from build123d import *

# Parameters (mm, degrees)
F0_W           = 40
F0_H           = 16
F1_DEPTH       = 12.7
F3_DEPTH       = 3.7
F4_R           = 6
F5_DEPTH       = 6
F6_R           = 8
F7_DEPTH       = 3
F9_D           = 5
F9_CBORE_D     = 9
F9_CBORE_DEPTH = 5


with BuildPart() as f1:
    # F0 (on Top) → F1 (new body)
    with BuildSketch(Plane.XY):
        Rectangle(F0_W, F0_H)
    extrude(amount=F1_DEPTH)

    # F2 (on face) → F3 (cut)
    with BuildSketch(Plane.XY.offset(12.7)):
        with BuildLine():
            ThreePointArc((-8, 8), (0, 0), (8, 8))
            Line((8, 8), (-8, 8))
        make_face()
    extrude(amount=-F3_DEPTH, mode=Mode.SUBTRACT)

    # F4 (on face) → F5 (cut)
    with BuildSketch(Plane.XY.offset(9)):
        with Locations((0, 8)):
            Circle(F4_R)
    extrude(amount=-F5_DEPTH, mode=Mode.SUBTRACT)

    # F6 (on face) → F7 (cut)
    with BuildSketch(Plane.XY.offset(3)):
        with Locations((0, 8)):
            Circle(F6_R)
    extrude(amount=-F7_DEPTH, mode=Mode.SUBTRACT)

    # F9 (through all)
    with Locations(Plane.XZ.offset(8)):
        with Locations((-13, 6), (13, 6)):
            CounterBoreHole(F9_D / 2, F9_CBORE_D / 2, F9_CBORE_DEPTH)


solid = f1.part
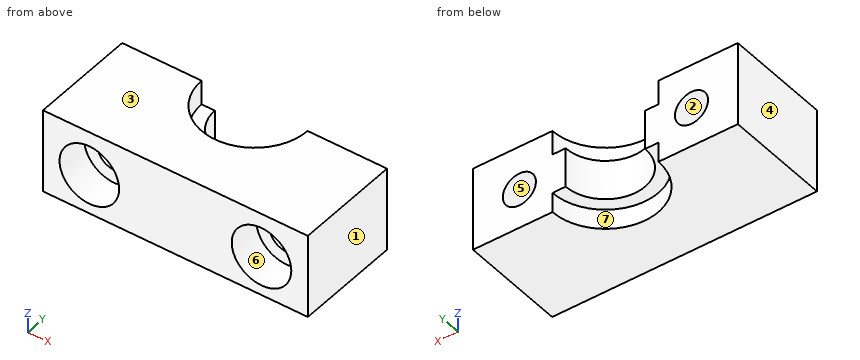
The listing builds one solid part. Answer for the finished solid, in the listing's coordinates (mm). Face numbers are marked on the shaded views. A direction names the side the tool comes from. Coordinates: 2 decimals unless noted, no trailing zeros. Order: outer loops, then holes, each group sorted by start corner. A loop starts at its lowest first (then second) coordinate and runs counter-clockwise, first axis right, second up.
Q1. Which of the six approach directions +Z, -Z, +X, -X, +Y, -Y give full straight-line access (tool end or side, diameter ignored) to the marked faces 5, 6 and 7?
Q2. A cutting plane is placed at A-A, the plane x = -13. Write down the section's boundary in (y, z).
Q3. A cutting plane is placed at D-D, the plane y = -4.25. Write down the section's boundary in (x, z), and give its area (3 significant figures).
Q4. For a pull along X with two mould halves and no side action, classify the marked faces 1, 2, 3 and 4 as pulls with the +X half, pulls with the -X half, needs draft (parallel to the pull), parting line crosses it, or undercut.
Q5. Given P1, Ø2.5, axis at x = 12.5, z = 6.5, coming from the -Y side; P2, Ø2, axis at x = 12.5, y = -3, coming from the -Z side; P3, Ø1.5, axis at x = -1.5, z = 10, coming from the +Y side; P4, Ø4.5, axis at x = -13.5, z = 5.5, coming from the -Y side, each flat-ended and moving along its own axis, determine where each tip first touches the part or whether it passes through.
Q6. A cutting plane is placed at C-C, the plane z = 6. Write down the section's boundary in (x, y), and give its area (3 significant figures).
Q7. A cutting plane is placed at B-B, the plane y = 5.75. Write down the section's boundary in (x, z).
Q8. Consider line 1 (Z direction, x = -13, y = 1.25); line 2 (Z direction, x = -13, y = -5.45); line 3 (X direction, y = 1.75, z = 6.25). Determine where each line is inside the solid, lowest interval first.
Answers follow:
1. face 5: +Y, -Y
1. face 6: -Y
1. face 7: -Z, +Y
2. outline: (-8, 0) - (8, 0) - (8, 3.5) - (-3, 3.5) - (-3, 1.5) - (-8, 1.5) - close; (-8, 10.5) - (-3, 10.5) - (-3, 8.5) - (8, 8.5) - (8, 12.7) - (-8, 12.7) - close
3. outline: (-20, 0) - (20, 0) - (20, 12.7) - (-20, 12.7) - close; hole circle Ø9 at (-13, 6); hole circle Ø9 at (13, 6)
3. area: 381 mm2
4. face 1: pulls with the +X half
4. face 2: undercut
4. face 3: needs draft
4. face 4: pulls with the -X half
5. P1: passes through
5. P2: stops at z = 0
5. P3: stops at y = 0.32
5. P4: stops at y = -3
6. outline: (-20, -8) - (-17.5, -8) - (-17.5, -3) - (-15.5, -3) - (-15.5, 8) - (-20, 8) - close; (-10.5, -3) - (-8.5, -3) - (-8.5, -8) - (8.5, -8) - (8.5, -3) - (10.5, -3) - (10.5, 8) - (6, 8) arc R6 cw to (-6, 8) - (-10.5, 8) - close; (15.5, -3) - (17.5, -3) - (17.5, -8) - (20, -8) - (20, 8) - (15.5, 8) - close
6. area: 383 mm2
7. outline: (-20, 0) - (-7.68, 0) - (-7.68, 3) - (-5.56, 3) - (-5.56, 9) - (-7.68, 9) - (-7.68, 12.7) - (-20, 12.7) - close; (5.56, 3) - (7.68, 3) - (7.68, 0) - (20, 0) - (20, 12.7) - (7.68, 12.7) - (7.68, 9) - (5.56, 9) - close; hole circle Ø5 at (-13, 6); hole circle Ø5 at (13, 6)
8. line 1: z = 0 to 3.5, 8.5 to 12.7
8. line 2: z = 0 to 1.5, 10.5 to 12.7
8. line 3: x = -20 to -15.49, -10.51 to 10.51, 15.49 to 20
